from build123d import *

# Parameters (mm, degrees)
BASE_FLANGE1_DEPTH = 6


# Sheet-metal steps are written as plain solids
with BuildPart() as part:
    # Sketch1 → Base-Flange1 (new body)
    with BuildSketch(Plane(origin=(0, 0, 0), x_dir=(0, 0, -1), z_dir=(1, 0, 0))):
        with BuildLine():
            Line((-31.859064644, 3), (-260, 3))
            Line((-260, 3), (-260, 18))
            Line((-260, 18), (-30, 80))
            Line((-30, 80), (30, 80))
            Line((30, 80), (410, 18))
            Line((410, 18), (410, 3))
            Line((410, 3), (31.859064644, 3))
            ThreePointArc((31.859064644, 3), (0, 32), (-31.859064644, 3))
        make_face()
    extrude(amount=-BASE_FLANGE1_DEPTH)


solid = part.part
The model under review builds one solid part; all positions refer to its coordinate system, in mm. Give positions to 0.01 mm unless a question says otherwise; leave off trailing zeros. Write each loop counter-clockwise with the first axis right and the second up, starting at its lowest first coordinate (ties: lowest second). Pieces come first, ordered by that corner, then holes.
1. Add section C-C, the plane y = 44.5. Write out the cut boundary in (x, z).
2. Add section A-A, the plane x = -4.2. Write out the cut boundary in (y, z), plus the area to 3 significant figures.
3. Draft analysis for pull direction Z (two halves, no side actions). For faces 1 (the flat face through (-2.958, 48.566, 146.61)), 2 (the flat face through (-2.958, 49.434, -217.34)), 3 (the cylindrical face through (-2.958, 31.993, -0.662)), state which applies: +Z half, -Z half, draft (parallel to the pull), parting line (faces both ways), or undercut.
4. Wall thickness on L1, parallel to Z at x = -1.2, y = 16; L2, parallel to Y at x = -4.6, z = -289.5; L3, parallel to Y at x = -3.45, z = 44.5: over which ranges is each line inside the solid? List them lowest first.
5. Add section B-B, the plane z = 3.5. Write out the cut boundary in (x, y).
6. For P1, Ø4, axis at y = 58, z = -69.5, coming from the +X side; P2, Ø2, axis at x = -1, z = -210, coming from the +Y side, all flat-tipped, find the tip position at first contact; note any pin that passes through.
Worked answers:
1. outline: (-6, -247.58) - (0, -247.58) - (0, 161.69) - (-6, 161.69) - close
2. outline: (3, -410) - (18, -410) - (80, -30) - (80, 30) - (18, 260) - (3, 260) - (3, 31.86) arc R32 cw to (3, -31.86) - close
2. area: 31,300 mm2
3. face 1: +Z half
3. face 2: -Z half
3. face 3: undercut
4. L1: z = -410 to -27.71, 27.71 to 260
4. L2: y = 3 to 37.66
4. L3: y = 3 to 76.09
5. outline: (-6, 31.81) - (0, 31.81) - (0, 80) - (-6, 80) - close
6. P1: stops at x = 0
6. P2: stops at y = 50.79
